Autodesk Inventor part; units mm, degrees
ref_plane "YZ Plane" through (0, 0, 0) normal (1, 0, 0) x (0, 1, 0)
ref_plane "XZ Plane" through (0, 0, 0) normal (0, 1, 0) x (-1, 0, 0)
ref_plane "XY Plane" through (0, 0, 0) normal (0, 0, 1) x (1, 0, 0)
sketch "Sketch1" plane through (0, 0, 0) normal (0, 1, 0) x (-1, 0, 0)
  line L0 (0, 0) -> (60, 0)
  line L1 (60, 0) -> (60, -60)
  line L2 (60, -60) -> (0, -60)
  line L3 (0, -60) -> (0, 0)
  circle A0 centre (51.2132, -8.7868) radius 2.25
  circle A1 centre (8.7868, -51.2132) radius 2.25
  circle A2 centre (8.7868, -8.7868) radius 2.25
  circle A3 centre (51.2132, -51.2132) radius 2.25
  line L4 (51.2132, -8.7868) -> (8.7868, -51.2132) construction
  line L5 (51.2132, -51.2132) -> (8.7868, -8.7868) construction
  line L6 (51.2132, -8.7868) -> (8.7868, -8.7868) construction
  line L7 (21, -24.5) -> (39, -24.5) construction
  line L8 (39, -24.5) -> (39, -35.5) construction
  line L9 (39, -35.5) -> (21, -35.5) construction
  line L10 (21, -35.5) -> (21, -24.5) construction
  line L11 (30, 0) -> (30, -60) construction
  circle A4 centre (21, -24.5) radius 1.75
  circle A5 centre (21, -35.5) radius 1.75
  line L12 (19, -22.5) -> (41, -22.5) construction
  line L13 (41, -22.5) -> (41, -52.5) construction
  line L14 (41, -52.5) -> (19, -52.5) construction
  line L15 (19, -52.5) -> (19, -22.5) construction
  line L16 (21, -24.5) -> (19, -24.5) construction
  line L17 (21, -24.5) -> (21, -22.5) construction
  line L18 (39, -24.5) -> (41, -24.5) construction
  circle A6 centre (39, -24.5) radius 1.75
  circle A7 centre (39, -35.5) radius 1.75
  arc A8 (24, -30) -> (36, -30) centre (30, -30) ccw
  line L19 (19, -52.5) -> (41, -52.5)
  line L20 (41, -52.5) -> (41, -38.5196)
  line L21 (41, -38.5196) -> (19, -38.5196)
  line L22 (19, -38.5196) -> (19, -52.5)
  circle A9 centre (21, -24.5) radius 2.5
  circle A10 centre (21, -35.5) radius 2.5
  circle A11 centre (39, -24.5) radius 2.5
  circle A12 centre (39, -35.5) radius 2.5
  line L23 (24, -30) -> (36, -30) construction
  line L24 (36, -30) -> (36, -22.75)
  line L25 (36, -22.75) -> (24, -22.75)
  line L26 (24, -22.75) -> (24, -30)
  line L27 (40.75, -26.2854) -> (40.75, -33.7146)
  line L28 (37.25, -33.7146) -> (37.25, -26.2854)
  line L29 (4, -16) -> (14, -16)
  line L30 (14, -16) -> (14, -44)
  line L31 (14, -44) -> (4, -44)
  line L32 (4, -44) -> (4, -16)
  line L33 (16, -4) -> (44, -4)
  line L34 (44, -4) -> (44, -14)
  line L35 (44, -14) -> (16, -14)
  line L36 (16, -14) -> (16, -4)
  line L37 (56, -16) -> (46, -16)
  line L38 (46, -16) -> (46, -44)
  line L39 (46, -44) -> (56, -44)
  line L40 (56, -44) -> (56, -16)
  point P0 (60, -30)
  point P1 (39, -30)
  point P2 (30, -24.5)
  dimension "d0" = 4.5
  dimension "d1" = 4.5
  dimension "d2" = 4.5
  dimension "d3" = 4.5
  dimension "d4" = 60
  dimension "d5" = 60
  dimension "d6" = 18
  dimension "d7" = 11
  dimension "d8" = 60
  dimension "d9" = 3.5
  dimension "d10" = 3.5
  dimension "d11" = 22
  dimension "d12" = 30
  dimension "d13" = 3.5
  dimension "d14" = 3.5
  dimension "d15" = 12
  dimension "d16" = 5
  dimension "d17" = 5
  dimension "d18" = 5
  dimension "d19" = 5
  dimension "d26" = 4
  dimension "d27" = 10
  dimension "d28" = 16
  dimension "d29" = 16
  dimension "d30" = 4
  dimension "d31" = 16
  dimension "d32" = 16
  dimension "d33" = 10
extrude "Extrusion1" add sketch "Sketch1" along normal blind 1 contours L0 L1 L2 L3
extrude "Extrusion2" add sketch "Sketch1" along normal blind 6 contours A9 | A10 | A11 | A12
fillet "Fillet1" radius 1 18 edges at (-41, 0.5, -52.5) (-41, 0.5, -38.5196) (-19, 0.5, -38.5196) (-19, 0.5, -52.5) (-36, 0.5, -22.75) (-24, 0.5, -22.75) (-44, 0.5, -4) (-44, 0.5, -14) (-56, 0.5, -44) (-56, 0.5, -16) (-46, 0.5, -44) (-46, 0.5, -16) (-16, 0.5, -4) (-16, 0.5, -14) (-4, 0.5, -44) (-4, 0.5, -16) (-14, 0.5, -16) (-14, 0.5, -44)
fillet "Fillet2" radius 5 4 edges at (0, 0.5, -60) (-60, 0.5, -60) (-60, 0.5, 0) (0, 0.5, 0)
properties part number "SensorMount_top"
Part model, mm, in its own coordinate system. A direction names the side the tool comes from. Coordinates: 2 decimals unless noted, no trailing zeros. Order: outer loops, then holes, each group sorted by start corner. A loop starts at its lowest first (then second) coordinate and runs counter-clockwise, first axis right, second up. Notation, with made-up numbers: (-3.75, -22.5) - (54.25, -22.5) arc R30 ccw to (54.25, 5.5) - close; hole circle Ø10 at (80.5, 79). An arc over 180 degrees is marked (long way). Return JSON: item names as keys, results as strings. Group by question number.
Item 1: Drill centre lines: probe 1 along Z at (x, y) = (-39, 2.8); probe 2 along X at (y, z) = (0.45, -51); probe 3 along X at (y, z) = (0.8, -42). Where is each one in solid material? Low to high. Write a range as from..to.
Item 2: Pull direction X, two halves, no side cores. Call faces 3 (the face through (-37, 6, -36)), 4 (the face through (-38.46, 3.62, -33.06)), 5 (the face through (-58.5, 0.51, -58.57)): pulls with the +X half, pulls with the -X half, needs draft (parallel to the pull), parting line crosses it, or undercut.
Item 3: Cut at B-B (x = -39). List the corners of the cut face in (y, z), plus the area to 3 significant figures.
Item 4: Cut at D-D (x = -21). List the corners of the cut face in (y, z).
Item 5: Pin check, flat tips, straight feed: pin 1 (1.5 mm diameter, centred on x = -30, y = 1.5, fed in from -Z); pin 2 (2 mm diameter, centred on x = -22.5, y = 5.5, fed in from -Z); pin 3 (6 mm diameter, centred on x = -51.21, z = -8.79, fed in from +Y). Stop position of each tip, or through.
Item 6: Which spindle directions (+Z, -Z, +X, -X, +Y, -Y) get a long thin tool onto all of the face, cutting with end or side? Do faces 1 (the face through (-18.5, 3.5, -35.6)), 2 (the face through (-19, 6, -25)). Say none if no direction does.
Item 7: Cut at C-C (y = 4.7). List the corners of the cut face in (x, z), plus the area to 3 significant figures.
Item 8: Cut at A-A (z = -24.5). State how many separate pieces and enclosed holes the cut face has, plus the area to 3 significant figures.
Check values:
{
 "1": {"probe 1": "z = -38..-37.25, -33.75..-33, -27..-26.25, -22.75..-22", "probe 2": "x = -60..-53.45, -48.97..-41, -19..-11.03, -6.55..0", "probe 3": "x = -60..-56, -46..-41, -19..-14, -4..0"},
 "2": {"face 3": "needs draft", "face 4": "undercut", "face 5": "pulls with the -X half"},
 "3": {"outline": "(0, -60) - (1, -60) - (1, -52.5) - (0, -52.5) - close; (0, -38.52) - (1, -38.52) - (1, -38) - (6, -38) - (6, -37.25) - (0, -37.25) - close; (0, -33.75) - (6, -33.75) - (6, -33) - (0, -33) - close; (0, -27) - (6, -27) - (6, -26.25) - (0, -26.25) - close; (0, -22.75) - (6, -22.75) - (6, -22) - (1, -22) - (1, -14) - (0, -14) - close; (0, -4) - (1, -4) - (1, 0) - (0, 0) - close", "area": "38.0 mm2"},
 "4": {"outline": "(0, -60) - (1, -60) - (1, -52.5) - (0, -52.5) - close; (0, -38.52) - (1, -38.52) - (1, -38) - (6, -38) - (6, -37.25) - (0, -37.25) - close; (0, -33.75) - (6, -33.75) - (6, -33) - (1, -33) - (1, -27) - (6, -27) - (6, -26.25) - (0, -26.25) - close; (0, -22.75) - (6, -22.75) - (6, -22) - (1, -22) - (1, -14) - (0, -14) - close; (0, -4) - (1, -4) - (1, 0) - (0, 0) - close"},
 "5": {"pin 1": "stops at z = -60", "pin 2": "stops at z = -37.95", "pin 3": "stops at y = 1"},
 "6": {"face 1": "+Y", "face 2": "+Z, -Z, +X, -X, +Y"},
 "7": {"outline": "circle Ø5 at (-39, -35.5); circle Ø5 at (-39, -24.5); circle Ø5 at (-21, -35.5); circle Ø5 at (-21, -24.5); hole circle Ø3.5 at (-39, -35.5); hole circle Ø3.5 at (-39, -24.5); hole circle Ø3.5 at (-21, -35.5); hole circle Ø3.5 at (-21, -24.5)", "area": "40.1 mm2"},
 "8": {"separate pieces": "6", "enclosed holes": "0", "area": "36.0 mm2"}
}
